Here's how the part is built. I have some questions about the finished solid (model axes, mm). A direction names the side the tool comes from. Round coordinates to 2 decimals unless told otherwise and drop trailing zeros. Order: outer loops, then holes, each group sorted by start corner. A loop starts at its lowest first (then second) coordinate and runs counter-clockwise, first axis right, second up. Notation, with made-up numbers: (78, 61) -> (116, 61) arc R36 ccw to (116, 95) -> close; hole circle Ø2 at (38, 21). An arc over 180 degrees is marked (long way). Use a Markdown table: item, result. Add a question column.
(1) I want a section at C-C, the plane y = 2. Please give me the cut outline in (x, z).
(2) I want a section at B-B, the plane x = 65. Please give me the cut outline in (y, z), then the cut area to 3 significant figures.
(3) On a 3-axis mill with a long thin cutter (end or side, diameter ignored), from which of +Z, -Z, +X, -X, +Y, -Y can I reach the whole of each face in a straight line? I mean faces 1 (the face through (5, 0, 5)), 2 (the face through (-80, -1, 6)), 3 (the face through (-28.554, -37.039, 2.535)). Say none if no direction works.
(4) If I drill on probe 1 along X at (y, z) = (0.5, 3.5); probe 2 along X at (y, z) = (-45, 9.5), over which ranges is the centre line in solid material (lowest first)?
(5) Thinking about a two-plate mould opening in X: for faces 4 (the face through (51.547, 68.979, 2.465)), 5 (the face through (-6, -77, 13)), 6 (the face through (80, -1, 6)), which applies, pulls with the +X half, pulls with the -X half, needs draft (parallel to the pull), parting line crosses it, or undercut?
(6) I want a section at A-A, the plane z = 8.5. Please give me the cut outline in (x, y), then the cut area to 3 significant figures.
(7) I'm going to push a flat-ended pin straight in: P1, Ø5, axis at x = 45, y = 41.5, coming from the +Z side. Where does the tip first touch, or does it pass through?
(8) I want a section at D-D, the plane x = -33.5. Please give me the cut outline in (y, z).
from build123d import *

# Parameters (mm, degrees)
SKETCH2_W           = 160
SKETCH2_H           = 160
BOSS_EXTRUDE1_DEPTH = 5
CUT_EXTRUDE1_REACH  = 115.248
SKETCH3_W           = 150
SKETCH3_H           = 150
BOSS_EXTRUDE2_DEPTH = 5
SKETCH5_W           = 160
SKETCH5_H           = 160
SKETCH5_W_2         = 150.5
SKETCH5_H_2         = 150.5
BOSS_EXTRUDE3_DEPTH = 8
FILLET1_R           = 10


with BuildPart() as part:
    # Sketch2 → Boss-Extrude1 (new body)
    with BuildSketch(Plane.XY):
        Rectangle(SKETCH2_W, SKETCH2_H)
    extrude(amount=BOSS_EXTRUDE1_DEPTH)

    # Sketch3 → Cut-Extrude1 (cut, up to next)
    with BuildSketch(Plane.XY.offset(5), mode=Mode.PRIVATE) as cut_extrude1_sk1:
        Rectangle(SKETCH3_W, SKETCH3_H)
    cut_extrude1_tool1 = extrude(cut_extrude1_sk1.sketch, amount=-CUT_EXTRUDE1_REACH, mode=Mode.PRIVATE) & part.part
    add(cut_extrude1_tool1.solids().sort_by_distance((0, 0, 5))[0], mode=Mode.SUBTRACT)

    # Sketch4 → Boss-Extrude2 (add)
    with BuildSketch(Plane.XY.offset(5)):
        Polygon((66.514718626, 75), (0, 8.485281374), (-66.514718626, 75), (-75, 75), (-75, 66.514718626), (-8.485281374, 0), (-75, -66.514718626), (-75, -75), (-66.514718626, -75), (0, -8.485281374), (66.514718626, -75), (75, -75), (75, -66.514718626), (8.485281374, 0), (75, 66.514718626), (75, 75), align=None)
    extrude(amount=-BOSS_EXTRUDE2_DEPTH)

    # Sketch5 → Boss-Extrude3 (add)
    with BuildSketch(Plane.XY.offset(5)):
        Rectangle(SKETCH5_W, SKETCH5_H)
        Rectangle(SKETCH5_W_2, SKETCH5_H_2, mode=Mode.SUBTRACT)
    extrude(amount=BOSS_EXTRUDE3_DEPTH)

    # Fillet1
    fillet1_edges = [part.edges().sort_by_distance(p)[0] for p in [
        (-66.514718626, 75, 2.5),
        (0, 8.485281374, 2.5),
        (66.514718626, 75, 2.5),
        (75, 66.514718626, 2.5),
        (8.485281374, 0, 2.5),
        (75, -66.514718626, 2.5),
        (66.514718626, -75, 2.5),
        (0, -8.485281374, 2.5),
        (-66.514718626, -75, 2.5),
        (-75, -66.514718626, 2.5),
        (-8.485281374, 0, 2.5),
        (-75, 66.514718626, 2.5),
    ]]
    fillet(fillet1_edges, radius=FILLET1_R)


solid = part.part
Taken from the geometry:
| question | item | result |
|---|---|---|
| 1 | outline | (-80, 0) -> (-75, 0) -> (-75, 5) -> (-75.25, 5) -> (-75.25, 13) -> (-80, 13) -> close; (-12.83, 0) -> (12.83, 0) -> (12.83, 5) -> (-12.83, 5) -> close; (75, 0) -> (80, 0) -> (80, 13) -> (75.25, 13) -> (75.25, 5) -> (75, 5) -> close |
| 2 | outline | (-80, 0) -> (-52.37, 0) -> (-52.37, 5) -> (-75.25, 5) -> (-75.25, 13) -> (-80, 13) -> close; (52.37, 0) -> (80, 0) -> (80, 13) -> (75.25, 13) -> (75.25, 5) -> (52.37, 5) -> close |
| 2 | area | 352 mm2 |
| 3 | face 1 | +Z |
| 3 | face 2 | +Z, -Z, -X, +Y, -Y |
| 3 | face 3 | +Z, -Z |
| 4 | probe 1 | x = -80 to -75, -12.64 to 12.64, 75 to 80 |
| 4 | probe 2 | x = -80 to -75.25, 75.25 to 80 |
| 5 | face 4 | undercut |
| 5 | face 5 | needs draft |
| 5 | face 6 | pulls with the +X half |
| 6 | outline | (-80, -80) -> (80, -80) -> (80, 80) -> (-80, 80) -> close; hole (-75.25, -75.25) -> (75.25, -75.25) -> (75.25, 75.25) -> (-75.25, 75.25) -> close |
| 6 | area | 2,950 mm2 |
| 7 | P1 | stops at z = 5 |
| 8 | outline | (-80, 0) -> (-75, 0) -> (-75, 5) -> (-75.25, 5) -> (-75.25, 13) -> (-80, 13) -> close; (-41.99, 0) -> (-25.01, 0) -> (-25.01, 5) -> (-41.99, 5) -> close; (25.01, 0) -> (41.99, 0) -> (41.99, 5) -> (25.01, 5) -> close; (75, 0) -> (80, 0) -> (80, 13) -> (75.25, 13) -> (75.25, 5) -> (75, 5) -> close |
